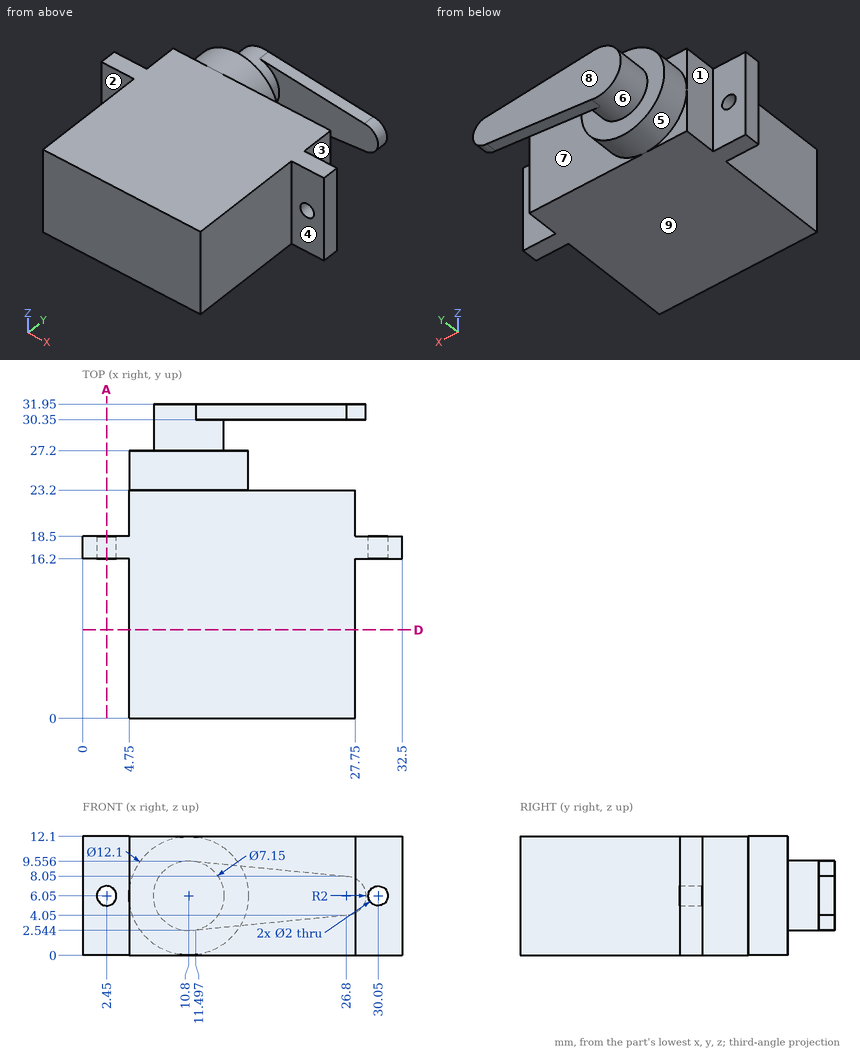
Geometry check sheet. Reference: drawing and pictorial views, mm from the part's lowest x, y, z. A direction names the side the tool comes from. Coordinates: 2 decimals unless noted, no trailing zeros. Write each loop counter-clockwise with the first axis right and the second up, starting at its lowest first coordinate (ties: lowest second). Pieces come first, ordered by that corner, then holes. Notation, with made-up numbers: M 9,12 L 45,12 A22 cw 45,45 Z; hole C -1,67.5 d7. An arc over 180 degrees is marked long. Use one line per item in the form item = value.
Item 1: Sectioned sample at A-A, the plane x = 2.45. Record the cut outline in (y, z).
Answer below:
outline = M 16.2,0 L 18.5,0 L 18.5,5.05 L 16.2,5.05 Z; M 16.2,7.05 L 18.5,7.05 L 18.5,12.1 L 16.2,12.1 Z
Item 2: Material ranges on L1, parallel to X at y = 17.1, z = 6.05; L2, parallel to Z at x = 30.05, y = 17.65; L3, parallel to Y at x = 20, z = 7.5, recorded low to high. Write a range as from..to.
Answer below:
L1 = 0..1.45, 3.45..29.05, 31.05..32.5
L2 = 0..5.05, 7.05..12.1
L3 = 0..23.2, 30.35..31.95
Item 3: Release check for a two-part mould opening along Y. For the marked faces 6, 7, 8 and 9 record: pulls with the +Y half, pulls with the -Y half, needs draft (parallel to the pull), parting line crosses it, or undercut.
Answer below:
face_6 = undercut
face_7 = undercut
face_8 = pulls with the +Y half
face_9 = needs draft
Item 4: Gauge pin test, flat ends, axial feed: pin 1 Ø6 at (y, z) = (19, 6) entering from +X; pin 2 Ø1.4 at (x, z) = (29.5, 6.5) entering from -Y; pin 3 Ø3 at (y, z) = (23.5, 9.5) entering from +X; pin 4 Ø3 at (y, z) = (26.5, 3.5) entering from -X. Record the tip position at first contact, or that the pin passes through.
Answer below:
pin_1 = 32.5
pin_2 = 16.2
pin_3 = 27.75
pin_4 = 4.84
Item 5: Set-up check for the marked faces 1, 2, 3, 4 and 5: record each of +Z, -Z, +X, -X, +Y, -Y from which the full face is reachable in a straight line by a thin tool's end or side.
Answer below:
face_1 = +Z, -Z, -X, +Y
face_2 = +Z, -Z, -X, -Y
face_3 = +Z, -Z, +X
face_4 = +Z, -Z, +X, -Y
face_5 = none
Item 6: Sectioned sample at D-D, the plane y = 9. Record the cut outline in (x, z), and give its area (3 significant figures).
Answer below:
outline = M 4.75,0 L 27.75,0 L 27.75,12.1 L 4.75,12.1 Z
area = 278 mm^2
